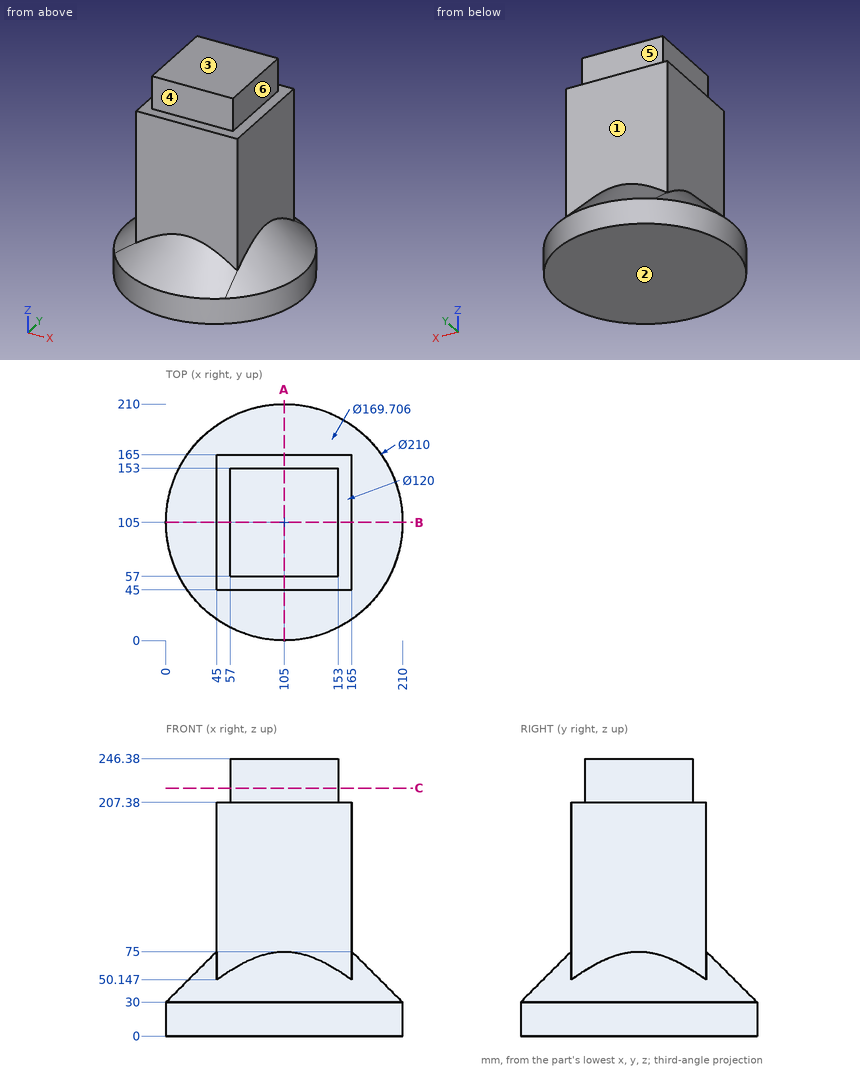
Source: three-view drawing plus pictorial views. Frame: mm from the lowest corner of the part. A direction names the side the tool comes from. Coordinates: 2 decimals unless noted, no trailing zeros. Order: outer loops, then holes, each group sorted by start corner. A loop starts at its lowest first (then second) coordinate and runs counter-clockwise, first axis right, second up. Notation, with made-up numbers: M -23.5,49 L -18.5,49 A33 ccw -18.5,78 Z; hole C -25.75,-9 d1. An arc over 180 degrees is marked long. One line per question, with ' | ' between items. Start each with the question number.
Item 1: Set-up query: the marked faces 4, 5 and 6. Return all of +Z, -Z, +X, -X, +Y, -Y with unobstructed straight access to the full face (end or side cutting, diameter ignored); none if empty.
Item 2: Cut plane C-C, the plane z = 220. Return the cut outline in (x, y), then the cut area to 3 significant figures.
Item 3: Ray query, probe 1 along Y at (x, z) = (150.5, 140.5); probe 2 along Z at (x, y) = (113.5, 51.5); probe 3 along X at (y, z) = (84, 233). Return the intervals inside material, ascending. Write a range as [from, to].
Item 4: Draft query along Z for the marked faces 1, 2 and 3. Return one class per face: released by +Z, released by -Z, zero draft, split by the parting line, or undercut.
Item 5: Cut plane A-A, the plane x = 105. Return the cut outline in (y, z).
Item 6: Pin query (flat end, axial travel): pin 1 Ø10 at (y, z) = (134.5, 84.5) entering from -X; pin 2 Ø5 at (x, z) = (89.5, 31.5) entering from -Y; pin 3 Ø5 at (x, z) = (120.5, 214) entering from +Y; pin 4 Ø3 at (x, z) = (167, 98.5) entering from +Y (3 decimals). Return the tip coordinate at first contact, or that it passes through.
A:
1) face 4: +Z, +X, -X, -Y | face 5: +Z, +X, -X, +Y | face 6: +Z, +X, +Y, -Y
2) outline: M 57,57 L 153,57 L 153,153 L 57,153 Z | area: 9,220 mm2
3) probe 1: y = [45, 165] | probe 2: z = [0, 207.38] | probe 3: x = [57, 153]
4) face 1: zero draft | face 2: released by -Z | face 3: released by +Z
5) outline: M 0,0 L 210,0 L 210,30 L 165,75 L 165,207.38 L 153,207.38 L 153,246.38 L 57,246.38 L 57,207.38 L 45,207.38 L 45,75 L 0,30 Z
6) pin 1: stops at x = 45 | pin 2: stops at y = 0.87 | pin 3: stops at y = 153 | pin 4: passes through
